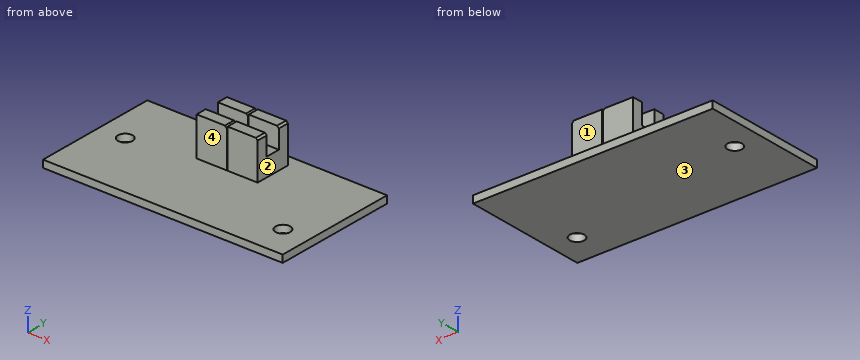
```python
from build123d import *

# Parameters (mm, degrees)
CROQUIS1_W              = 33
CROQUIS1_H              = 17.2
CROQUIS1_R              = 1
SALIENTE_EXTRUIR1_DEPTH = 1
CROQUIS2_W              = 8.4
CROQUIS2_H              = 5
SALIENTE_EXTRUIR2_DEPTH = 2.5
CROQUIS2_5_W            = 8.4
CROQUIS2_5_H            = 1.5
SALIENTE_EXTRUIR3_DEPTH = 5.3
CORTAR_EXTRUIR1_START   = -5.3
CROQUIS3_W              = 0.1
CROQUIS3_H              = 5
CORTAR_EXTRUIR1_DEPTH   = 5.3
CHAFL_N1_SIZE           = 0.25


with BuildPart() as part:
    # Croquis1 → Saliente-Extruir1 (new body)
    with BuildSketch(Plane.XY):
        Rectangle(CROQUIS1_W, CROQUIS1_H)
        with Locations((-12.9, 0.65)):
            Circle(CROQUIS1_R, mode=Mode.SUBTRACT)
        with Locations((12.9, -4.25)):
            Circle(CROQUIS1_R, mode=Mode.SUBTRACT)
    extrude(amount=SALIENTE_EXTRUIR1_DEPTH)

    # Croquis2 → Saliente-Extruir2 (add)
    with BuildSketch(Plane.XY.offset(1)):
        with Locations((0, 4.5)):
            Rectangle(CROQUIS2_W, CROQUIS2_H)
    extrude(amount=SALIENTE_EXTRUIR2_DEPTH)

    # Croquis2<5> → Saliente-Extruir3 (add)
    with BuildSketch(Plane.XY.offset(1)):
        with Locations((0, 2.75)):
            Rectangle(CROQUIS2_5_W, CROQUIS2_5_H)
        with Locations((0, 6.25)):
            Rectangle(CROQUIS2_5_W, CROQUIS2_5_H)
    extrude(amount=SALIENTE_EXTRUIR3_DEPTH)

    # Croquis3 → Cortar-Extruir1 (cut)
    with BuildSketch(Plane.XY.offset(6.3).offset(CORTAR_EXTRUIR1_START)):
        with Locations((0, 4.5)):
            Rectangle(CROQUIS3_W, CROQUIS3_H)
    extrude(amount=CORTAR_EXTRUIR1_DEPTH, mode=Mode.SUBTRACT)

    # Chaflán1
    chafl_n1_edges = [part.edges().sort_by_distance(p)[0] for p in [
        (4.2, 2.75, 6.3),
        (4.2, 6.25, 6.3),
        (-0.05, 2.75, 6.3),
        (-0.05, 6.25, 6.3),
    ]]
    chamfer(chafl_n1_edges, length=CHAFL_N1_SIZE)


solid = part.part
```
Build history of the part. All positions in model axes, mm. Face numbers are marked on the shaded views. A direction names the side the tool comes from. Round coordinates to 2 decimals unless told otherwise and drop trailing zeros. Write each loop counter-clockwise with the first axis right and the second up, starting at its lowest first coordinate (ties: lowest second). Pieces come first, ordered by that corner, then holes.
1) 3-axis set-ups, long thin cutter, end or side, ignore diameter. For the marked faces 1, 2, 3 and 4: which of +Z, -Z, +X, -X, +Y, -Y reach the whole face in a straight line?
2) Band-saw the part on D-D, the plane x = -3.5. List the corners of the cut face in (y, z).
3) Band-saw the part on A-A, the plane z = 5.25. List the corners of the cut face in (x, y).
4) Band-saw the part on B-B, the plane y = -4.25. List the corners of the cut face in (x, z), and give its area (3 significant figures).
5) Drill centre lines: probe 1 along Y at (x, z) = (-12.9, 0.8); probe 2 along Y at (x, z) = (12.9, 0.4); probe 3 along Z at (x, y) = (-8, 2). Where is each one in solid material? Low to high.
6) Pin check, flat tips, straight feed: pin 1 (2.5 mm diameter, centred on x = 12.9, y = -4.25, fed in from +Z); pin 2 (1.4 mm diameter, centred on x = -1, z = 5, fed in from +Y); pin 3 (1.5 mm diameter, centred on y = 5.5, z = 2.5, fed in from +X). Stop position of each tip, or through.
7) Band-saw the part on C-C, the plane x = 13.5. List the corners of the cut face in (y, z), and give its area (3 significant figures).
Ans:
1. face 1: +Z, +X, -X, +Y
1. face 2: +Z, +X, +Y, -Y
1. face 3: -Z, +X, -X, +Y, -Y
1. face 4: +Z, +X, -X, -Y
2. outline: (-8.6, 0) - (8.6, 0) - (8.6, 1) - (7, 1) - (7, 6.3) - (5.5, 6.3) - (5.5, 3.5) - (3.5, 3.5) - (3.5, 6.3) - (2, 6.3) - (2, 1) - (-8.6, 1) - close
3. outline: (-4.2, 2) - (-0.05, 2) - (-0.05, 3.5) - (-4.2, 3.5) - close; (-4.2, 5.5) - (-0.05, 5.5) - (-0.05, 7) - (-4.2, 7) - close; (0.05, 2) - (4.2, 2) - (4.2, 3.5) - (0.05, 3.5) - close; (0.05, 5.5) - (4.2, 5.5) - (4.2, 7) - (0.05, 7) - close
4. outline: (-16.5, 0) - (11.9, 0) - (11.9, 1) - (-16.5, 1) - close; (13.9, 0) - (16.5, 0) - (16.5, 1) - (13.9, 1) - close
4. area: 31.0 mm2
5. probe 1: y = -8.6 to -0.35, 1.65 to 8.6
5. probe 2: y = -8.6 to -5.25, -3.25 to 8.6
5. probe 3: z = 0 to 1
6. pin 1: stops at z = 1
6. pin 2: stops at y = 7
6. pin 3: stops at x = 4.2
7. outline: (-8.6, 0) - (-5.05, 0) - (-5.05, 1) - (-8.6, 1) - close; (-3.45, 0) - (8.6, 0) - (8.6, 1) - (-3.45, 1) - close
7. area: 15.6 mm2
